Input: part model. Units: mm. Frame: model coordinates. A direction names the side the tool comes from. Coordinates: 2 decimals unless noted, no trailing zeros. Write each loop counter-clockwise with the first axis right and the second up, starting at its lowest first coordinate (ties: lowest second). Pieces come first, ordered by that corner, then holes. Notation, with made-up numbers: (10.5, 57) -> (42.5, 57) arc R14 cw to (42.5, 78) -> close; hole circle Ø4 at (12, 44.5). An arc over 180 degrees is marked (long way). One line per question, with ' | ' between items. Start each with the question number.
```python
from build123d import *

# Parameters (mm, degrees)
BOSS_EXTRUDE1_DEPTH = 6.35
CUT_EXTRUDE1_REACH  = 13.714
SKETCH2_R           = 2
FILLET1_SIZE        = 0.4


with BuildPart() as part:
    # Sketch1 → Boss-Extrude1 (new body)
    with BuildSketch(Plane.XY):
        with BuildLine():
            Line((-11.5951, -2.938456882), (-11.5951, 2.938456882))
            Line((-11.5951, 2.938456882), (-11.539212407, 2.938456882))
            ThreePointArc((-11.539212407, 2.938456882), (-10.585316586, 3.333573468), (-10.1902, 4.287469289))
            Line((-10.1902, 4.287469289), (-10.1902, 6.402089023))
            ThreePointArc((-10.1902, 6.402089023), (-9.74154152, 7.073969797), (-8.94902056, 6.917034355))
            Line((-8.94902056, 6.917034355), (-5.652895046, 3.628441884))
            ThreePointArc((-5.652895046, 3.628441884), (-5.027976112, 2.694919539), (-4.8085, 1.593185507))
            Line((-4.8085, 1.593185507), (-4.8085, -1.593185507))
            ThreePointArc((-4.8085, -1.593185507), (-5.027976112, -2.694919539), (-5.652895046, -3.628441884))
            Line((-5.652895046, -3.628441884), (-8.94902056, -6.917034355))
            ThreePointArc((-8.94902056, -6.917034355), (-9.74154152, -7.073969797), (-10.1902, -6.402089023))
            Line((-10.1902, -6.402089023), (-10.1902, -4.287469289))
            ThreePointArc((-10.1902, -4.287469289), (-10.585316586, -3.333573468), (-11.539212407, -2.938456882))
            Line((-11.539212407, -2.938456882), (-11.5951, -2.938456882))
        make_face()
    extrude(amount=BOSS_EXTRUDE1_DEPTH)

    # Sketch2 → Cut-Extrude1 (cut, up to next)
    with BuildSketch(Plane.ZY.offset(11.5951), mode=Mode.PRIVATE) as cut_extrude1_sk1:
        with Locations((3.175, 0)):
            Circle(SKETCH2_R)
    cut_extrude1_tool1 = extrude(cut_extrude1_sk1.sketch, amount=-CUT_EXTRUDE1_REACH, mode=Mode.PRIVATE) & part.part
    add(cut_extrude1_tool1.solids().sort_by_distance((-11.5951, 0, 3.175))[0], mode=Mode.SUBTRACT)

    # Fillet1
    fillet1_edges = [part.edges().sort_by_distance(p)[0] for p in [
        (-11.5951, 0, 1.175),
    ]]
    chamfer(fillet1_edges, length=FILLET1_SIZE)


solid = part.part
```
1) Section D-D, the plane x = -9.5. Return loops of the section in (y, z) (3 decimals).
2) Section C-C, the plane x = -10.5. Return loops of the section in (y, z) (3 decimals), then the cut area to 3 significant figures.
3) Pull-direction query (Z, two-part tool) for faces 4 (the face through (-8, 0, 6.35)), 5 (the face through (-8.05, -0.77, 5.02)), 6 (the face through (-4.808, 0, 6)); classes: released by +Z, released by -Z, zero draft, split by the parting line, or undercut.
4) Ray query, line 1 (Y direction, x = -10.5, z = 3.5); line 2 (Y direction, x = -8.25, z = 2.75); line 3 (Z direction, x = -5.75, y = -0.5). Return the intervals inside material, ascending.
5) Access query for faces 1 (the face through (-10.19, -5, 3)), 2 (the face through (-10.19, 5, 3)), 3 (the face through (-8, 0, 0)). Directions: +Z, -Z, +X, -X, +Y, -Y. A direction counts if a zero-diameter tool reaches every point of the face in a straight line with its end or side. Return the directions, or none.
6) First-contact query: P1, Ø0.6, axis at y = -5, z = 4.5, coming from the -X side; P2, Ø2.5, axis at y = 5, z = 3, coming from the -X side; P3, Ø1.5, axis at x = -8.5, z = 1, coming from the -Y side. Flat tips, straight axial feed; report the tip coordinate or a pass-through.
Answer block:
1) outline: (-7.129, 0) -> (7.129, 0) -> (7.129, 6.35) -> (-7.129, 6.35) -> close; hole circle Ø4 at (0, 3.175)
2) outline: (-3.427, 0) -> (3.427, 0) -> (3.427, 6.35) -> (-3.427, 6.35) -> close; hole circle Ø4 at (0, 3.175) | area: 31.0 mm2
3) face 4: released by +Z | face 5: undercut | face 6: zero draft
4) line 1: y = -3.43 to -1.97, 1.97 to 3.43 | line 2: y = -6.22 to -1.95, 1.95 to 6.22 | line 3: z = 0 to 1.24, 5.11 to 6.35
5) face 1: +Z, -Z, -X, -Y | face 2: +Z, -Z, -X, +Y | face 3: -Z, +X, -X, +Y, -Y
6) P1: stops at x = -10.19 | P2: stops at x = -10.3 | P3: stops at y = -7.1
